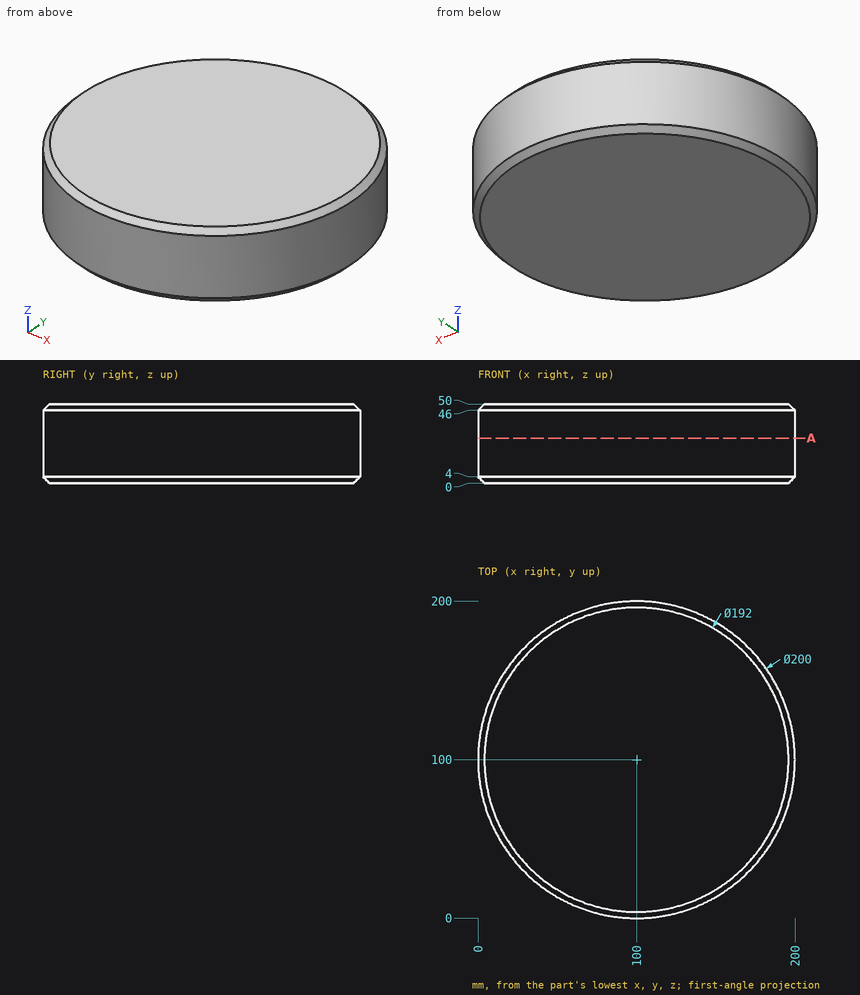
For this review, use the dimensioned drawing (mm, ordinates from the lowest corner) and the shaded views. Coordinates: 2 decimals unless noted, no trailing zeros. Loops run counter-clockwise (first coordinate to the right, second up) from the corner with the lowest first, then second, coordinate; pieces in that order, holes last. Notation, with made-up numbers: (55, -13.75) -> (75, -13.75) arc R14 ccw to (75, 9.25) -> close; hole circle Ø1 at (1.5, -11.75). An arc over 180 degrees is marked (long way). Use a Markdown table: item, result. Add a question column.
Item 1: Clearance check with flat-ended pins moving along their axes: P1, Ø4, axis at x = 72.5, z = 38, coming from the +Y side; P2, Ø10, axis at y = 139.5, z = 22, coming from the +X side; P3, Ø1.5, axis at y = 26, z = 39.5, coming from the +X side. State where each tip first meets the part, or that it passes through.
Item 2: We need section A-A, the plane z = 28.5. Write out the cut boundary in (x, y).
Item 3: Wall thickness on L1, parallel to X at y = 128.5, z = 37.5; L2, parallel to Y at x = 160, z = 23.5; L3, parallel to Y at x = 13, z = 5: over which ranges is each line inside the solid? List them lowest first. Write a range as from..to.
Numbers:
| question | item | result |
|---|---|---|
| 1 | P1 | stops at y = 196.69 |
| 1 | P2 | stops at x = 193.86 |
| 1 | P3 | stops at x = 168.08 |
| 2 | outline | circle Ø200 at (100, 100) |
| 3 | L1 | x = 4.15..195.85 |
| 3 | L2 | y = 20..180 |
| 3 | L3 | y = 50.69..149.31 |
